The drawing under review shows one solid part. Ordinate dimensions are in mm from its lowest x, y, z. A direction names the side the tool comes from. Coordinates: 2 decimals unless noted, no trailing zeros. Order: outer loops, then holes, each group sorted by start corner. A loop starts at its lowest first (then second) coordinate and runs counter-clockwise, first axis right, second up. Notation, with made-up numbers: (27.25, -19.75) - (69.25, -19.75) arc R26 cw to (69.25, 11.25) - close; hole circle Ø8 at (76, -22.75). An arc over 180 degrees is marked (long way). Answer in a Markdown table with one row per item.
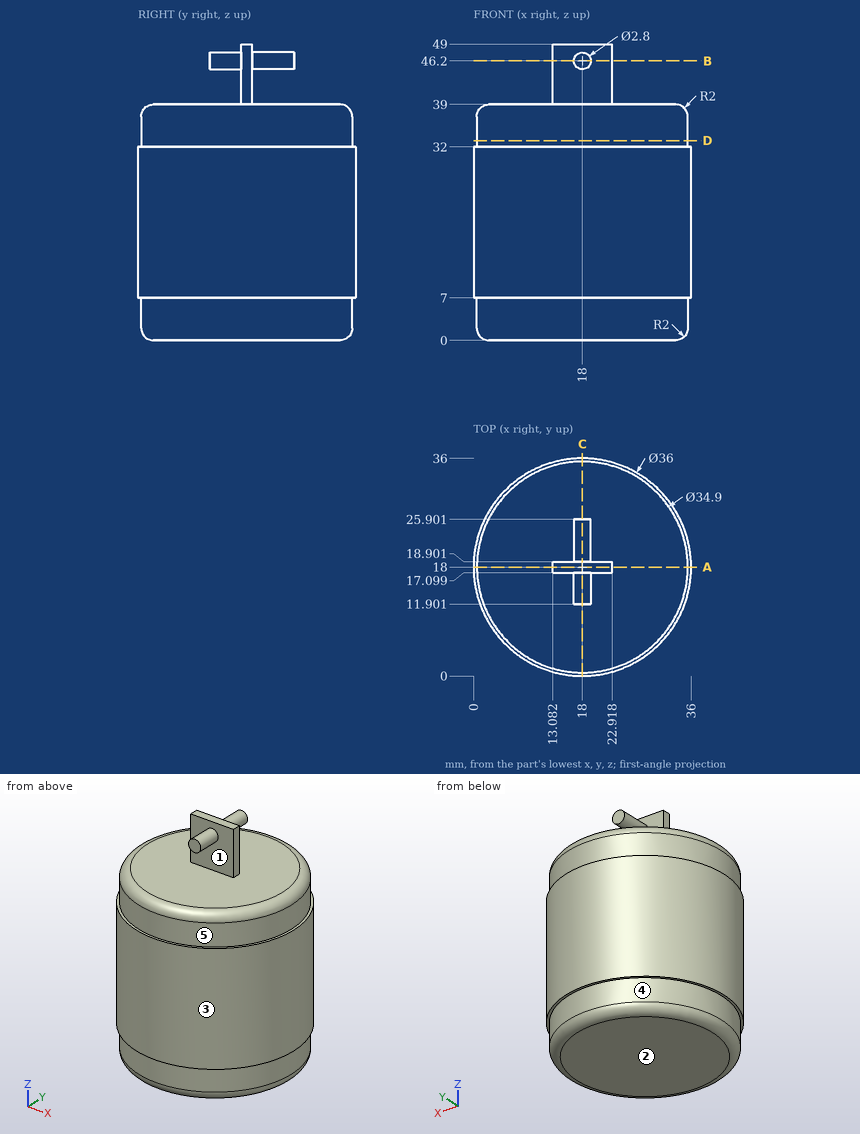
Item 1: We need section B-B, the plane z = 46.2. Write out the cut boundary in (x, y).
Check values:
| item | result |
|---|---|
| outline | (13.08, 17.1) - (16.6, 17.1) - (16.6, 11.9) - (19.4, 11.9) - (19.4, 17.1) - (22.92, 17.1) - (22.92, 18.9) - (19.4, 18.9) - (19.4, 25.9) - (16.6, 25.9) - (16.6, 18.9) - (13.08, 18.9) - close |
Item 2: To check wall thickness, follow line 1 (Z direction, x = 12, y = 25); line 2 (Z direction, x = 18.5, y = 20); line 3 (X direction, y = 31, z = 24). State the ranges of each line that lie inside material, in increasing order. Write a range as from..to.
Check values:
| item | result |
|---|---|
| line 1 | 0..39 |
| line 2 | 0..39, 44.89..47.51 |
| line 3 | 5.55..30.45 |
Item 3: Clearance check with flat-ended pins moving along their axes: pin 1 Ø3 at (x, z) = (20, 42.5) entering from -Y; pin 2 Ø3 at (x, z) = (18.5, 45.5) entering from +Y; pin 3 Ø1.5 at (x, z) = (12, 10.5) entering from +Y. State where each tip first meets the part, or that it passes through.
Check values:
| item | result |
|---|---|
| pin 1 | y = 17.1 |
| pin 2 | y = 25.9 |
| pin 3 | y = 35.22 |
Item 4: Tool access review of the marked faces 4 and 5: name each direction out of +Z, -Z, +X, -X, +Y, -Y from which nothing blocks a thin tool from reaching the whole face with its end or side.
Check values:
| item | result |
|---|---|
| face 4 | -Z |
| face 5 | +Z |
Item 5: We need section A-A, the plane y = 18. Write out the cut boundary in (x, z).
Check values:
| item | result |
|---|---|
| outline | (0, 7) - (0.55, 7) - (0.55, 2) arc R2 ccw to (2.55, 0) - (33.45, 0) arc R2 ccw to (35.45, 2) - (35.45, 7) - (36, 7) - (36, 32) - (35.45, 32) - (35.45, 37) arc R2 ccw to (33.45, 39) - (22.92, 39) - (22.92, 49) - (13.08, 49) - (13.08, 39) - (2.55, 39) arc R2 ccw to (0.55, 37) - (0.55, 32) - (0, 32) - close |
Item 6: Mouldability with a two-part tool opening along Z and no side actions: class the marked faces 1, 2 and 3 as +Z half, -Z half, draft (parallel to the pull), parting line (faces both ways), or undercut.
Check values:
| item | result |
|---|---|
| face 1 | undercut |
| face 2 | -Z half |
| face 3 | draft |
Item 7: We need section D-D, the plane z = 33. Write out the cut boundary in (x, y), then the cut area to 3 significant figures.
Check values:
| item | result |
|---|---|
| outline | circle Ø34.9 at (18, 18) |
| area | 957 mm^2 |
Item 8: We need section C-C, the plane x = 18. Write out the cut boundary in (y, z), then the cut area to 3 significant figures.
Check values:
| item | result |
|---|---|
| outline | (0, 7) - (0.55, 7) - (0.55, 2) arc R2 ccw to (2.55, 0) - (33.45, 0) arc R2 ccw to (35.45, 2) - (35.45, 7) - (36, 7) - (36, 32) - (35.45, 32) - (35.45, 37) arc R2 ccw to (33.45, 39) - (18.9, 39) - (18.9, 44.8) - (25.9, 44.8) - (25.9, 47.6) - (18.9, 47.6) - (18.9, 49) - (17.1, 49) - (17.1, 47.6) - (11.9, 47.6) - (11.9, 44.8) - (17.1, 44.8) - (17.1, 39) - (2.55, 39) arc R2 ccw to (0.55, 37) - (0.55, 32) - (0, 32) - close |
| area | 1,440 mm^2 |
